from build123d import *

# Parameters (mm, degrees)
SKETCH1_R           = 7
BOSS_EXTRUDE1_DEPTH = 12
SKETCH3_R           = 2.5
SKETCH4_R           = 7
SKETCH5_R           = 2.5
BOSS_EXTRUDE2_DEPTH = 14
SKETCH6_R           = 4
CUT_EXTRUDE1_DEPTH  = 14


with BuildPart() as part:
    # Sketch1 → Boss-Extrude1 (new body)
    with BuildSketch(Plane(origin=(0, 0, 0), x_dir=(1, 0, 0), z_dir=(0, 1, 0))):
        with Locations(Location((0, 0, 0), (0, 0, 270))):
            Circle(SKETCH1_R)
    extrude(amount=BOSS_EXTRUDE1_DEPTH)

    # Sketch3 → Loft1 section 0
    with BuildSketch(Plane(origin=(0, 20, 0), x_dir=(1, 0, 0), z_dir=(0, 1, 0))):
        Circle(SKETCH3_R)
    # Sketch4 → Loft1 section 1
    with BuildSketch(Plane(origin=(0, 12, 0), x_dir=(1, 0, 0), z_dir=(0, 1, 0))):
        Circle(SKETCH4_R)
    loft()

    # Sketch5 → Boss-Extrude2 (add)
    with BuildSketch(Plane(origin=(0, 20, 0), x_dir=(1, 0, 0), z_dir=(0, 1, 0))):
        with Locations(Location((0, 0, 0), (0, 0, 270))):
            Circle(SKETCH5_R)
    extrude(amount=BOSS_EXTRUDE2_DEPTH)

    # Sketch6 → Cut-Extrude1 (cut)
    with BuildSketch(Plane.XZ):
        with Locations(Location((0, 0, 0), (0, 0, 270))):
            Circle(SKETCH6_R)
    extrude(amount=-CUT_EXTRUDE1_DEPTH, mode=Mode.SUBTRACT)


solid = part.part
Geometry: final body of the model. Coordinates: model frame, mm. A direction names the side the tool comes from. Give positions to 0.01 mm unless a question says otherwise; leave off trailing zeros. Loops run counter-clockwise (first coordinate to the right, second up) from the corner with the lowest first, then second, coordinate; pieces in that order, holes last. Notation, with made-up numbers: M 8,46.25 L 58,46.25 A15 cw 58,72.25 Z; hole C 19,-2 d11. An arc over 180 degrees is marked long. Put each result on its own line as item: value.
1) Mould query, pull axis Z, two halves, no side actions, for faces 4 (the flat face through (-3, 0, 3)), 5 (the flat face through (0, 14, 0)), 6 (the conical face through (3.607, 17.722, -1.136)). Classes: released by +Z, released by -Z, zero draft, split by the parting line, or undercut.
Computed values:
face 4: zero draft
face 5: undercut
face 6: split by the parting line
2) Cut plane B-B, the plane y = 9.5. Return the cut outline in (x, z).
Computed values:
outline: C 0,0 d14; hole C 0,0 d8
3) Reachability of faces 1 (the cylindrical face through (-3.905, 6.902, 0.867)), 2 (the flat face through (0, 34, 0)), 3 (the cylindrical face through (-2.44, 26.9, -0.54)) from +Z, -Z, +X, -X, +Y, -Y: full face, straight path, thin tool, end or side. Return the list, or none.
Computed values:
face 1: -Y
face 2: +Z, -Z, +X, -X, +Y
face 3: +Y
4) Material intervals for L1, parallel to X at y = 8.25, z = 0; L2, parallel to Y at x = 0.25, z = -0.75; L3, parallel to Z at x = 3, y = 4, sorted ascending. Write a range as from..to.
Computed values:
L1: x = -7..-4, 4..7
L2: y = 14..34
L3: z = -6.32..-2.65, 2.65..6.32
5) First-contact query: P1, Ø1.5, axis at y = 24, z = -0.5, coming from the +X side; P2, Ø2.5, axis at x = -0.5, z = 1.5, coming from the -Y side; P3, Ø1.5, axis at x = 2.5, y = 19, coming from the -Z side. Flat tips, straight axial feed; report the tip coordinate or a pass-through.
Computed values:
P1: stops at x = 2.5
P2: stops at y = 14
P3: stops at z = -2.72
6) Cut plane D-D, the plane y = 17.5. Return the cut outline in (x, z).
Computed values:
outline: C 0,0 d7.81
7) Cut plane A-A, the plane x = 0. Return the cut outline in (y, z).
Computed values:
outline: M 0,-7 L 12,-7 L 20,-2.5 L 34,-2.5 L 34,2.5 L 20,2.5 L 12,7 L 0,7 L 0,4 L 14,4 L 14,-4 L 0,-4 Z
8) Cut plane C-C, the plane y = 26.5. Return the cut outline in (x, z), plus the area to 3 significant figures.
Computed values:
outline: C 0,0 d5
area: 19.6 mm^2
